```python
from build123d import *

# Parameters (mm, degrees)
SKETCH001_R  = 28.5
PAD_DEPTH    = 8
SKETCH_R     = 26.65
POCKET_DEPTH = 6
FILLET_R     = 1


with BuildPart() as part:
    # Sketch001 → Pad (new body)
    with BuildSketch(Plane.XY):
        Circle(SKETCH001_R)
    extrude(amount=PAD_DEPTH)

    # Sketch → Pocket (cut)
    with BuildSketch(Plane.XY):
        Circle(SKETCH_R)
    extrude(amount=POCKET_DEPTH, mode=Mode.SUBTRACT)

    # Fillet
    fillet_edges = [part.edges().sort_by_distance(p)[0] for p in [
        (-28.5, 0, 8),
        (-28.5, 0, 0),
        (-26.65, 0, 6),
    ]]
    fillet(fillet_edges, radius=FILLET_R)


solid = part.part
```
The model under review builds one solid part; all positions refer to its coordinate system, in mm. Give positions to 0.01 mm unless a question says otherwise; leave off trailing zeros. Write each loop counter-clockwise with the first axis right and the second up, starting at its lowest first coordinate (ties: lowest second). Pieces come first, ordered by that corner, then holes. Notation, with made-up numbers: M 76,39 L 87,39 A25 ccw 87,52 Z; hole C -31,-37.75 d10. An arc over 180 degrees is marked long. Write item = value, one per line. Start each with the question number.
Q1. For line 1 (Y direction, x = 0, z = 1.6); line 2 (Z direction, x = 4.5, y = 10); line 3 (X direction, y = 19, z = 2.5), list the stretches that pass through material, from the lowest coordinate up.
Q2. We need section A-A (y = 0). State the section outline as (x, z) points, plus the area to 3 significant figures.
Q3. We need section C-C (z = 2.75). State the section outline as (x, y) points.
Q4. Mouldability with a two-part tool opening along Y and no side actions: class faces 1 (the face through (-5.777, -26.016, 2.465)), 2 (the face through (0, 0, 6)), 3 (the face through (26.327, -10.916, 3.958)), 4 (the face through (0, 0, 8)) as released by +Y, released by -Y, zero draft, split by the parting line, or undercut.
Q5. Clearance check with flat-ended pins moving along their axes: pin 1 (6 mm diameter, centred on x = -3, y = -1.5, fed in from -Z); pin 2 (1 mm diameter, centred on x = -11, z = 6.5, fed in from -Y); pin 3 (1 mm diameter, centred on x = 2, z = 3.5, fed in from -Y). State where each tip first meets the part, or that it passes through.
Result set:
q1.line_1 = -28.5 to -26.65, 26.65 to 28.5
q1.line_2 = 6 to 8
q1.line_3 = -21.24 to -18.69, 18.69 to 21.24
q2.outline = M -28.5,1 A1 ccw -27.5,0 L -26.65,0 L -26.65,5 A1 cw -25.65,6 L 25.65,6 A1 cw 26.65,5 L 26.65,0 L 27.5,0 A1 ccw 28.5,1 L 28.5,7 A1 ccw 27.5,8 L -27.5,8 A1 ccw -28.5,7 Z
q2.area = 136 mm2
q3.outline = C 0,0 d57; hole C 0,0 d53.3
q4.face_1 = undercut
q4.face_2 = undercut
q4.face_3 = split by the parting line
q4.face_4 = zero draft
q5.pin_1 = 6
q5.pin_2 = -26.5
q5.pin_3 = -28.46
